Answer from the drawing. Dimensions are ordinates in mm from the lowest x, y and z of the part. Give positions to 0.01 mm unless a question says otherwise; leave off trailing zeros. Write each loop counter-clockwise with the first axis right and the second up, starting at its lowest first coordinate (ties: lowest second). Pieces come first, ordered by that corner, then holes. Notation, with made-up numbers: M -30.75,77.5 L 7.25,77.5 A22 cw 7.25,89.5 Z; hole C 53.25,40 d11. An arc over 180 degrees is marked long. Answer as a JSON object with one key per item and string values.
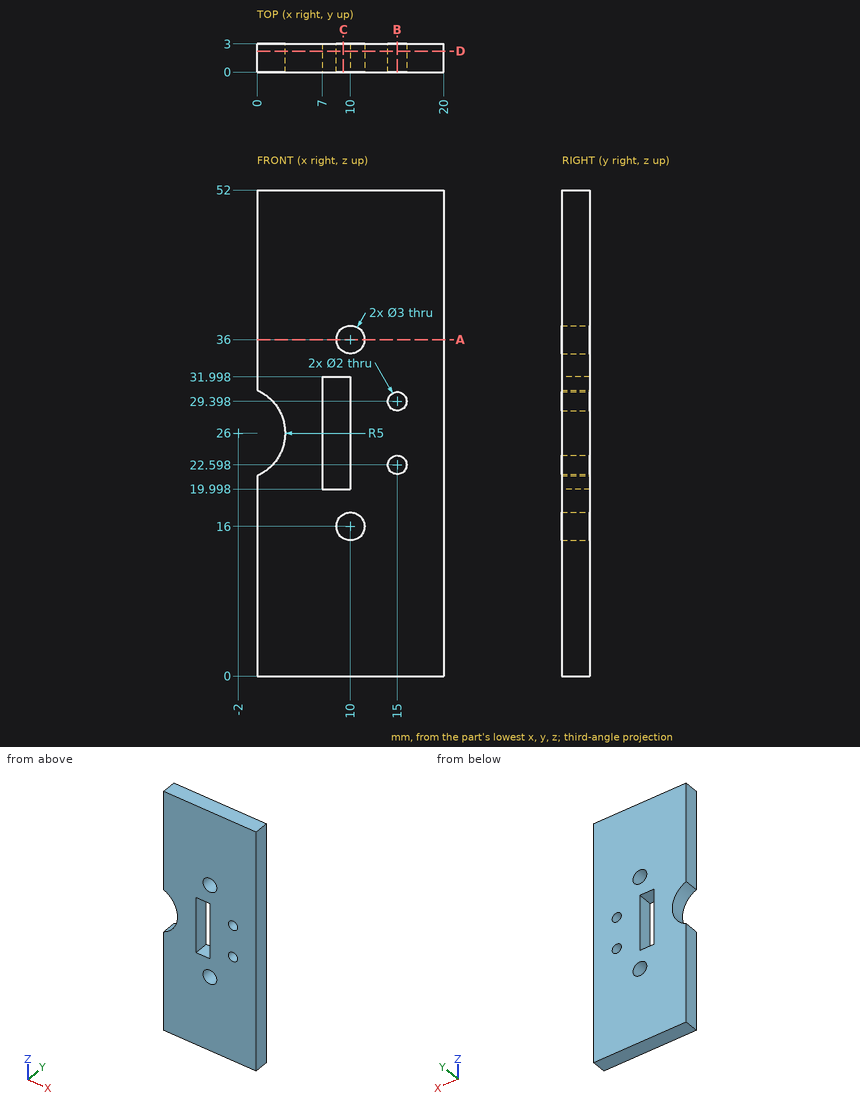
1. Consider line 1 along Z through (x, y) = (15, 0.95); line 2 along X through (y, z) = (1.8, 16); line 3 along Z through (x, y) = (10.5, 0.75) (1 decimal). Determine where each line is inside the solid, lowest interval first.
Verdict:
{"line 1": "z = 0 to 21.6, 23.6 to 28.4, 30.4 to 52", "line 2": "x = 0 to 8.5, 11.5 to 20", "line 3": "z = 0 to 14.6, 17.4 to 34.6, 37.4 to 52"}
2. A cutting plane is placed at C-C, the plane x = 9.25. Give the vertices of the cut face in (y, z), plus the area to 3 significant figures.
Verdict:
{"outline": "M 0,0 L 3,0 L 3,14.7 L 0,14.7 Z; M 0,17.3 L 3,17.3 L 3,20 L 0,20 Z; M 0,32 L 3,32 L 3,34.7 L 0,34.7 Z; M 0,37.3 L 3,37.3 L 3,52 L 0,52 Z", "area": "104 mm2"}
3. A cutting plane is placed at D-D, the plane y = 2.25. Give the vertices of the cut face in (x, z).
Verdict:
{"outline": "M 0,0 L 20,0 L 20,52 L 0,52 L 0,30.58 A5 cw 0,21.42 Z; hole M 7,20 L 10,20 L 10,32 L 7,32 Z; hole C 10,16 d3; hole C 10,36 d3; hole C 15,22.6 d2; hole C 15,29.4 d2"}
4. A cutting plane is placed at B-B, the plane x = 15. Give the vertices of the cut face in (y, z).
Verdict:
{"outline": "M 0,0 L 3,0 L 3,21.6 L 0,21.6 Z; M 0,23.6 L 3,23.6 L 3,28.4 L 0,28.4 Z; M 0,30.4 L 3,30.4 L 3,52 L 0,52 Z"}
5. A cutting plane is placed at A-A, the plane z = 36. Give the vertices of the cut face in (x, y).
Verdict:
{"outline": "M 0,0 L 8.5,0 L 8.5,3 L 0,3 Z; M 11.5,0 L 20,0 L 20,3 L 11.5,3 Z"}
